```python
from build123d import *

# Parameters (mm, degrees)
RESSALTO_EXTRUS_O1_DEPTH         = 1.25
ESBO_O5_W                        = 11.5
ESBO_O5_H                        = 7
CORTE_EXTRUS_O1_DEPTH            = 2.5
PADR_O_LINEAR1_COUNT             = 3
PADR_O_LINEAR1_PITCH             = 9
ESBO_O8_W                        = 11.5
ESBO_O8_H                        = 7
CORTE_EXTRUS_O4_DEPTH            = 10
PADR_O_LINEAR3_COUNT             = 3
PADR_O_LINEAR3_PITCH             = 11.5
ESPELHAR1_COPY_1_SKETCH_W        = 11.5
ESPELHAR1_COPY_1_SKETCH_H        = 7
ESPELHAR1_COPY_1_DEPTH           = 10
ESPELHAR1_COPY_2_SKETCH_W        = 11.5
ESPELHAR1_COPY_2_SKETCH_H        = 7
ESPELHAR1_COPY_2_DEPTH           = 10
ESPELHAR2_COPY_1_SKETCH_W        = 11.5
ESPELHAR2_COPY_1_SKETCH_H        = 7
ESPELHAR2_COPY_1_DEPTH           = 2.5
ESPELHAR2_COPY_2_SKETCH_W        = 11.5
ESPELHAR2_COPY_2_SKETCH_H        = 7
ESPELHAR2_COPY_2_DEPTH           = 2.5
CORTE_EXTRUS_O5_DEPTH            = 10
ESBO_O10_R                       = 1.75
RESSALTO_EXTRUS_O2_DEPTH         = 0.9
ESBO_O11_R                       = 2.5
ESBO_O11_R_2                     = 1.75
RESSALTO_EXTRUS_O3_DEPTH         = 1.5
PADR_O_LINEAR4_COUNT             = 2
PADR_O_LINEAR4_PITCH             = 38
PADR_O_LINEAR4_COUNT_DIR2        = 2
PADR_O_LINEAR4_PITCH_DIR2        = 16
PADR_O_LINEAR4_COPY_1_SKETCH_R   = 2.5
PADR_O_LINEAR4_COPY_1_SKETCH_R_2 = 1.75
PADR_O_LINEAR4_COPY_1_DEPTH      = 1.5
ESPELHAR5_COPY_1_SKETCH_R        = 2.5
ESPELHAR5_COPY_1_SKETCH_R_2      = 1.75
ESPELHAR5_COPY_1_DEPTH           = 1.5


with BuildPart() as part:
    # Esboço1 → Ressalto-extrusão1 (new body, symmetric)
    with BuildSketch(Plane(origin=(0, 0, 0), x_dir=(1, 0, 0), z_dir=(0, 1, 0))):
        Polygon((-24.393815238, -54.2), (-9.15, -54.2), (10.553192421, -30.65), (10.553192421, 30.65), (-9.15, 54.2), (-24.393815238, 54.2), (-22.610275313, 21), (-8, 21), (-8, -21), (-22.610275313, -21), align=None)
    extrude(amount=RESSALTO_EXTRUS_O1_DEPTH, both=True)

    # Esboço5 → Corte-extrusão1 (cut)
    with BuildSketch(Plane(origin=(0, 1.25, 0), x_dir=(1, 0, 0), z_dir=(0, 1, 0))):
        with Locations((3.624348025, -4.75)):
            Rectangle(ESBO_O5_W, ESBO_O5_H)
    corte_extrus_o1 = extrude(amount=-CORTE_EXTRUS_O1_DEPTH, mode=Mode.SUBTRACT)

    # Padrão linear1: Corte-extrusão1 ×3
    with Locations(*[(0, 0, i * PADR_O_LINEAR1_PITCH) for i in range(1, PADR_O_LINEAR1_COUNT)]):
        add(corte_extrus_o1, mode=Mode.SUBTRACT)

    # Esboço8 → Corte-extrusão4 (cut)
    with BuildSketch(Plane(origin=(0, 1.25, 0), x_dir=(1, 0, 0), z_dir=(0, 1, 0))):
        with Locations((-15.36, 26.27)):
            Rectangle(ESBO_O8_W, ESBO_O8_H)
    corte_extrus_o4 = extrude(amount=-CORTE_EXTRUS_O4_DEPTH, mode=Mode.SUBTRACT)

    # Padrão linear3: Corte-extrusão4 ×3
    with Locations(*[(0, 0, -i * PADR_O_LINEAR3_PITCH) for i in range(1, PADR_O_LINEAR3_COUNT)]):
        add(corte_extrus_o4, mode=Mode.SUBTRACT)

    # Espelhar1: Corte-extrusão4 across plane
    add(corte_extrus_o4.mirror(Plane.XY), mode=Mode.SUBTRACT)

    # Espelhar1 copy 1 sketch → Espelhar1 copy 1 (cut)
    with BuildSketch(Plane(origin=(0, 1.25, 11.5), x_dir=(1, 0, 0), z_dir=(0, 1, 0))):
        with Locations((-15.36, -26.27)):
            Rectangle(ESPELHAR1_COPY_1_SKETCH_W, ESPELHAR1_COPY_1_SKETCH_H)
    extrude(amount=-ESPELHAR1_COPY_1_DEPTH, mode=Mode.SUBTRACT)

    # Espelhar1 copy 2 sketch → Espelhar1 copy 2 (cut)
    with BuildSketch(Plane(origin=(0, 1.25, 23), x_dir=(1, 0, 0), z_dir=(0, 1, 0))):
        with Locations((-15.36, -26.27)):
            Rectangle(ESPELHAR1_COPY_2_SKETCH_W, ESPELHAR1_COPY_2_SKETCH_H)
    extrude(amount=-ESPELHAR1_COPY_2_DEPTH, mode=Mode.SUBTRACT)

    # Espelhar2: Corte-extrusão1 across plane
    add(corte_extrus_o1.mirror(Plane.XY), mode=Mode.SUBTRACT)

    # Espelhar2 copy 1 sketch → Espelhar2 copy 1 (cut)
    with BuildSketch(Plane(origin=(0, 1.25, -9), x_dir=(1, 0, 0), z_dir=(0, 1, 0))):
        with Locations((3.624348025, 4.75)):
            Rectangle(ESPELHAR2_COPY_1_SKETCH_W, ESPELHAR2_COPY_1_SKETCH_H)
    extrude(amount=-ESPELHAR2_COPY_1_DEPTH, mode=Mode.SUBTRACT)

    # Espelhar2 copy 2 sketch → Espelhar2 copy 2 (cut)
    with BuildSketch(Plane(origin=(0, 1.25, -18), x_dir=(1, 0, 0), z_dir=(0, 1, 0))):
        with Locations((3.624348025, 4.75)):
            Rectangle(ESPELHAR2_COPY_2_SKETCH_W, ESPELHAR2_COPY_2_SKETCH_H)
    extrude(amount=-ESPELHAR2_COPY_2_DEPTH, mode=Mode.SUBTRACT)

    # Esboço9 → Corte-extrusão5 (cut)
    with BuildSketch(Plane(origin=(0, 1.25, 0), x_dir=(1, 0, 0), z_dir=(0, 1, 0))):
        Polygon((8.455719459, -29.435601452), (-7.375936588, -28.25205491), (-6.609249814, -47.710896474), align=None)
    corte_extrus_o5 = extrude(amount=-CORTE_EXTRUS_O5_DEPTH, mode=Mode.SUBTRACT)

    # Espelhar3: Corte-extrusão5 across plane
    add(corte_extrus_o5.mirror(Plane.XY), mode=Mode.SUBTRACT)

    # Esboço10 → Ressalto-extrusão2 (add, symmetric)
    with BuildSketch(Plane(origin=(0, 0, 0), x_dir=(1, 0, 0), z_dir=(0, 1, 0))):
        with BuildLine():
            Line((-28.61, -33.75), (-23.29521911, -33.75))
            Line((-23.29521911, -33.75), (-23.751848307, -42.25))
            Line((-23.751848307, -42.25), (-28.61, -42.25))
            ThreePointArc((-28.61, -42.25), (-32.86, -38), (-28.61, -33.75))
        make_face()
        with Locations((-28.61, -38)):
            Circle(ESBO_O10_R, mode=Mode.SUBTRACT)
    ressalto_extrus_o2 = extrude(amount=RESSALTO_EXTRUS_O2_DEPTH, both=True)

    # Esboço11 → Ressalto-extrusão3 (add)
    with BuildSketch(Plane(origin=(0, 0.9, 0), x_dir=(1, 0, 0), z_dir=(0, 1, 0))):
        with Locations((-28.61, -38)):
            Circle(ESBO_O11_R)
        with Locations((-28.61, -38)):
            Circle(ESBO_O11_R_2, mode=Mode.SUBTRACT)
    ressalto_extrus_o3 = extrude(amount=RESSALTO_EXTRUS_O3_DEPTH)

    # Espelhar4: Ressalto-extrusão3 across plane
    add(ressalto_extrus_o3.mirror(Plane.ZX))

    # Padrão linear4: Ressalto-extrusão2, Ressalto-extrus_o3 2 × 2, 2 skipped
    with Locations(*[(j * PADR_O_LINEAR4_PITCH_DIR2, 0, -i * PADR_O_LINEAR4_PITCH) for i in range(PADR_O_LINEAR4_COUNT) for j in range(PADR_O_LINEAR4_COUNT_DIR2) if (i, j) not in ((0, 0), (0, 1), (1, 0))]):
        add(ressalto_extrus_o2)
        add(ressalto_extrus_o3)

    # Padrão linear4 copy 1 sketch → Padrão linear4 copy 1 (add)
    with BuildSketch(Plane(origin=(16, -0.9, -38), x_dir=(1, 0, 0), z_dir=(0, -1, 0))):
        with Locations((-28.61, 38)):
            Circle(PADR_O_LINEAR4_COPY_1_SKETCH_R)
        with Locations((-28.61, 38)):
            Circle(PADR_O_LINEAR4_COPY_1_SKETCH_R_2, mode=Mode.SUBTRACT)
    extrude(amount=PADR_O_LINEAR4_COPY_1_DEPTH)

    # Espelhar5: Ressalto-extrusão3, Ressalto-extrusão2 across plane
    add(ressalto_extrus_o3.mirror(Plane.XY))
    add(ressalto_extrus_o2.mirror(Plane.XY))

    # Espelhar5 copy 1 sketch → Espelhar5 copy 1 (add)
    with BuildSketch(Plane.XZ.offset(0.9)):
        with Locations((-28.61, -38)):
            Circle(ESPELHAR5_COPY_1_SKETCH_R)
        with Locations((-28.61, -38)):
            Circle(ESPELHAR5_COPY_1_SKETCH_R_2, mode=Mode.SUBTRACT)
    extrude(amount=ESPELHAR5_COPY_1_DEPTH)


solid = part.part
```
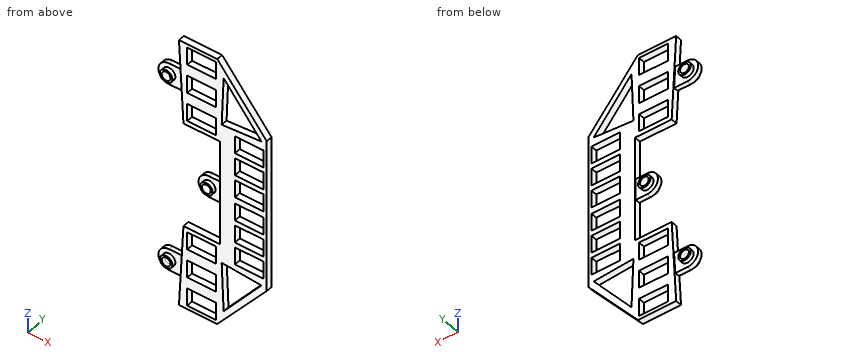
Part model, mm, in its own coordinate system. Coordinates: 2 decimals unless noted, no trailing zeros. Order: outer loops, then holes, each group sorted by start corner. A loop starts at its lowest first (then second) coordinate and runs counter-clockwise, first axis right, second up. Notation, with made-up numbers: (88.25, -36) - (144.25, -36) arc R19 cw to (144.25, -10) - close; hole circle Ø3 at (-33, -5). An arc over 180 degrees is marked (long way). Return JSON: item names as keys, results as strings. Group by question number.
Item 1: Cut at A-A (z = 0). List the corners of the cut face in (x, y), plus the area to 3 significant figures.
Item 2: Cut at B-B (z = 38). List the corners of the cut face in (x, y), plus the area to 3 significant figures.
Item 3: Pin check, flat tips, straight feed: pin 1 (4 mm diameter, centred on x = -11.5, z = -11.5, fed in from -Y); pin 2 (0.8 mm diameter, centred on y = 0.5, z = -37.5, fed in from +X); pin 3 (1.5 mm diameter, centred on x = -9, z = -24, fed in from +Y); pin 4 (1.2 mm diameter, centred on x = 6, y = -0.5, fed in from +Z). Stop position of each tip, or through.
Item 4: Drill centre lines: probe 1 along Z at (x, y) = (-28.61, 0.55); probe 2 along Z at (x, y) = (-9.5, -0.1); probe 3 along Z at (x, y) = (-28.61, -1.35). Where is each one in solid material? Low to high. Write a range as from..to.
Item 5: Cut at C-C (y = -0.05). State how many separate pieces and enclosed holes the cut face has, plus the area to 3 significant figures.
Check values:
{
 "1": {"outline": "(-16.86, -0.9) - (-15.11, -0.9) - (-15.11, -2.4) - (-14.36, -2.4) - (-14.36, 2.4) - (-15.11, 2.4) - (-15.11, 0.9) - (-16.86, 0.9) - close; (-10.86, -2.4) - (-10.11, -2.4) - (-10.11, -0.9) - (-8, -0.9) - (-8, -1.25) - (10.55, -1.25) - (10.55, 1.25) - (-8, 1.25) - (-8, 0.9) - (-10.11, 0.9) - (-10.11, 2.4) - (-10.86, 2.4) - close", "area": "60.5 mm2"},
 "2": {"outline": "(-32.86, -0.9) - (-31.11, -0.9) - (-31.11, -2.4) - (-30.36, -2.4) - (-30.36, 2.4) - (-31.11, 2.4) - (-31.11, 0.9) - (-32.86, 0.9) - close; (-26.86, -2.4) - (-26.11, -2.4) - (-26.11, -0.9) - (-23.52, -0.9) - (-23.52, -1.25) - (-21.11, -1.25) - (-21.11, 1.25) - (-23.52, 1.25) - (-23.52, 0.9) - (-26.11, 0.9) - (-26.11, 2.4) - (-26.86, 2.4) - close; (-9.61, -1.25) - (-6.99, -1.25) - (-6.99, 1.25) - (-9.61, 1.25) - close; (1.4, -1.25) - (4.4, -1.25) - (4.4, 1.25) - (1.4, 1.25) - close", "area": "35.1 mm2"},
 "3": {"pin 1": "passes through", "pin 2": "stops at x = 5.16", "pin 3": "stops at y = 1.25", "pin 4": "stops at z = 36.81"},
 "4": {"probe 1": "z = -42.25..-39.75, -36.25..-33.75, 33.75..36.25, 39.75..42.25", "probe 2": "z = -54.2..-21, -4.25..4.25, 21..54.2", "probe 3": "z = -40.5..-39.75, -36.25..-35.5, 35.5..36.25, 39.75..40.5"},
 "5": {"separate pieces": "1", "enclosed holes": "17", "area": "1,490 mm2"}
}
